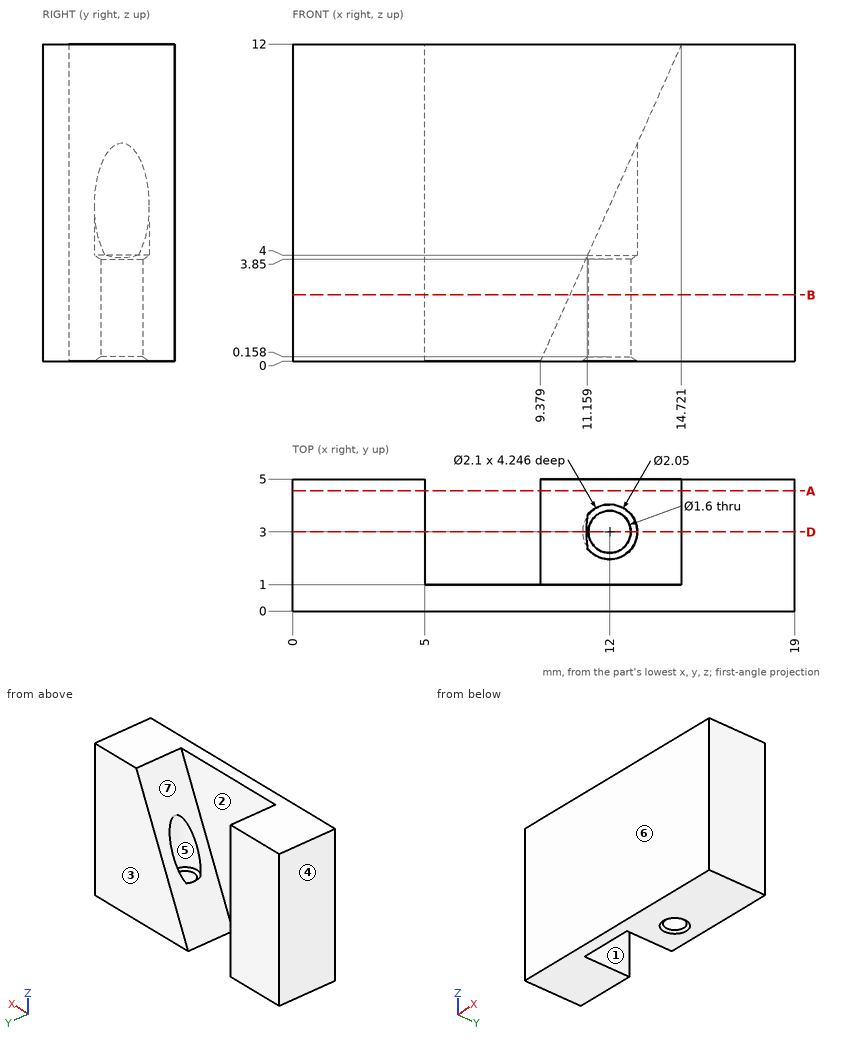
Answer from the drawing. Dimensions are ordinates in mm from the lowest x, y and z of the part. A direction names the side the tool comes from. Give positions to 0.01 mm unless a question says otherwise; leave off trailing zeros. Order: outer loops, then holes, each group sorted by start corner. A loop starts at its lowest first (then second) coordinate and runs counter-clockwise, first axis right, second up. Notation, with made-up numbers: (-8, 33) -> (16, 33) arc R8 ccw to (16, 45) -> close; hole circle Ø10 at (-23, -2). An arc over 180 degrees is marked (long way). One line per item, written item: value.
Item 1: A flat-ended cylindrical pin translates along its axis: P1, Ø2, axis at x = 12, y = 3, coming from the +Z side. Find the tip coordinate at first contact, or state that the pin passes through.
Answer sheet:
P1: z = 3.97
Item 2: Determine the mould class of the marked faces 1, 2, 3 and 4 for opening direction X: released by +X, released by -X, zero draft, split by the parting line, or undercut.
Answer sheet:
face 1: undercut
face 2: undercut
face 3: zero draft
face 4: released by -X
Item 3: Find section A-A, the plane y = 4.55. Give the vertices of the cut face in (x, z).
Answer sheet:
outline: (0, 0) -> (5, 0) -> (5, 12) -> (0, 12) -> close; (9.38, 0) -> (19, 0) -> (19, 12) -> (14.72, 12) -> close
Item 4: Find section B-B, the plane z = 2.5. Give the vertices of the cut face in (x, y).
Answer sheet:
outline: (0, 0) -> (19, 0) -> (19, 5) -> (10.49, 5) -> (10.49, 1) -> (5, 1) -> (5, 5) -> (0, 5) -> close; hole circle Ø1.6 at (12, 3)
Item 5: Find section D-D, the plane y = 3. State how many separate pieces and enclosed holes the cut face has, plus the area to 3 significant figures.
Answer sheet:
separate pieces: 3
enclosed holes: 0
area: 133 mm²
Item 6: A tool of negligible diameter and unlimited length cuts with its end or side. For the marked faces 5, 6 and 7, from which of +Z, -Z, +X, -X, +Y, -Y can it reach the whole face along a straight path? Write none if from no direction.
Answer sheet:
face 5: +Z
face 6: +Z, -Z, +X, -X, -Y
face 7: +Z, +Y
Item 7: Straight lines are drawn through the part: probe 1 along X at (y, z) = (3, 5.2); probe 2 along Y at (x, z) = (12, 1.4); probe 3 along Y at (x, z) = (12, 4.95). For each, find the intervals that lie inside material, in ascending order.
Answer sheet:
probe 1: 0 to 5, 13.05 to 19
probe 2: 0 to 2.2, 3.8 to 5
probe 3: 0 to 1.95, 4.05 to 5
